CAD build for the part. Positions are in the model's coordinates, mm. A direction names the side the tool comes from. Give positions to 0.01 mm unless a question says otherwise; leave off trailing zeros. Loops run counter-clockwise (first coordinate to the right, second up) from the corner with the lowest first, then second, coordinate; pieces in that order, holes last. Notation, with made-up numbers: (-22.5, 24.5) -> (-1.5, 24.5) arc R25 cw to (-1.5, 50.5) -> close; hole circle Ø2 at (9, 82.5). An arc over 180 degrees is marked (long way). Write each question's results on one line, items separated by ' | '. Start each with the question number.
Autodesk Inventor part; units mm, degrees
ref_plane "YZ Plane" through (0, 0, 0) normal (1, 0, 0) x (0, 1, 0)
ref_plane "XZ Plane" through (0, 0, 0) normal (0, 1, 0) x (-1, 0, 0)
ref_plane "XY Plane" through (0, 0, 0) normal (0, 0, 1) x (1, 0, 0)
sketch "Sketch1" plane through (0, 0, 0) normal (0, 1, 0) x (-1, 0, 0)
  line L0 (22.75, -10.36) -> (7.75, -10.36)
  line L1 (7.75, -10.36) -> (-0.1031, 0)
  circle A0 centre (4.34, -10.36) radius 1
  line L2 (22.75, 10.36) -> (7.75, 10.36)
  circle A1 centre (12.64, 0) radius 9.6 construction
  line L3 (22.75, 12.36) -> (22.75, -12.36)
  circle A2 centre (4.34, 10.36) radius 1
  line L4 (7.75, 10.36) -> (-0.1031, 0)
  line L5 (26.25, 19) -> (26.25, -19)
  line L6 (22.75, -12.36) -> (-22.75, -12.36)
  line L7 (22.75, 0) -> (-22.75, 0) construction
  line L8 (26.25, -19) -> (-28.75, -19)
  line L9 (26.25, -19) -> (-28.75, 19) construction
  line L10 (-28.75, -19) -> (26.25, 19) construction
  line L11 (-22.75, 12.36) -> (22.75, 12.36)
  line L12 (-28.75, 19) -> (26.25, 19)
  line L13 (-28.75, -19) -> (-28.75, 19)
  circle A3 centre (-16.36, 10.25) radius 1
  line L14 (-22.75, -12.36) -> (-22.75, 12.36)
  circle A4 centre (-16.36, -10.25) radius 1
  point P0 (0, 0)
  point P1 (-1.25, 0)
  point P2 (0, 0)
  point P3 (22.75, -10.36)
  dimension "d0" = 55
  dimension "d1" = 38
  dimension "d2" = 45.5
  dimension "d3" = 24.72
  dimension "d4" = 2
  dimension "d6" = 18.41
  dimension "d7" = 20.5
  dimension "d8" = 19.2
  dimension "d9" = 10.11
  dimension "d10" = 13
  dimension "d11" = 15
  dimension "d12" = 3.5
  dimension "d13" = 2
  dimension "d14" = 3.41
  dimension "d66" = 20.7
extrude "Extrusion1" add sketch "Sketch1" along normal mid plane 1 contours L3 L6 L14 L11 L2 L4 L1 L0 | L5 L8 L13 L12
extrude "Extrusion2" add sketch "Sketch1" along normal blind 35 contours L5 L8 L13 L12
fillet "Fillet1" radius 3 8 edges at (1.25, -0.5, -19) (28.75, -0.5, 0) (1.25, -0.5, 19) (-26.25, -0.5, 0) (28.75, 17.25, -19) (28.75, 17.25, 19) (-26.25, 17.25, 19) (-26.25, 17.25, -19)
sketch "Sketch5" plane through (25.75, 2.5, -19) normal (0, 0, -1) x (-1, 0, 0)
  circle A0 centre (2.5, 14.75) radius 1.5
  circle A1 centre (2.5, 21.75) radius 1.5
  circle A2 centre (2.5, 28.75) radius 1.5
  circle A3 centre (16.5, 14.75) radius 1.5
  circle A4 centre (16.5, 21.75) radius 1.5
  circle A5 centre (16.5, 28.75) radius 1.5
  line L0 (-3, 32.5) -> (-3, 0)
  line L1 (0, 32.5) -> (49, 32.5)
  point P0 (25.75, -2.5)
  dimension "d47" = 3
  dimension "d52" = 7
  dimension "d55" = 14
  dimension "d67" = 3.75
  dimension "d68" = 5.5
hole "Hole2" at (23.25, 17.25, -19) at (23.25, 24.25, -19) at (9.25, 24.25, -19) at (9.25, 17.25, -19) at (23.25, 31.25, -19) at (9.25, 31.25, -19) direction (0, 0, 1) diameter 2.459 depth 6 tip angle 118 counterbore diameter 3.9 counterbore depth 3.8
sketch "Sketch8" plane through (0, 35, 0) normal (0, 1, 0) x (1, 0, 0)
  line L0 (-23.25, -19) -> (25.75, -19)
  line L1 (28.75, -16) -> (28.75, 16)
  point P0 (0, 0)
  point P1 (16.25, -15.68)
  dimension "d77" = 3.32
  dimension "d78" = 12.5
hole "Hole4" at (16.25, 35, 15.68) direction (0, -1, 0) diameter 2.459 depth 6 tip angle 118 counterbore diameter 3.9 counterbore depth 3.8
properties part number "basketlewy" material "PCTG 20%"
Q1. Which spindle directions (+Z, -Z, +X, -X, +Y, -Y) get a long thin tool onto all of the face, cutting with end or side? Do faces 1 (the face through (9.2, 22.3, -17.1)), 2 (the face through (22.75, 18, 0)), 3 (the face through (0.91, 0.36, 18.1)). Say none if no direction does.
Q2. Drop flat-ended pins along their axis: pin 1 (4.5 mm diameter, centred on x = 8.5, y = 17.5, fed in from -Z); pin 2 (6 mm diameter, centred on x = 9, z = 2, fed in from +Y); pin 3 (1.5 mm diameter, centred on x = 23.25, y = 24.25, fed in from -Z); pin 4 (1.9 mm diameter, centred on x = 23.5, y = 32, fed in from -Z). Give the stop position or say it passes through.
Q3. Mould opens along Y. For faces 4 (the face through (9.998, 30.274, -14.085)), 5 (the face through (7, -0.5, 0)), 6 (the face through (17.98, 33.07, 16.58)) say: pulls with the +Y half, pulls with the -Y half, needs draft (parallel to the pull), parting line crosses it, or undercut.
Q4. Wall check: L1, parallel to X at y = 31.25, z = -13.95; L2, parallel to Z at x = -15, y = 28; L3, parallel to Y at x = 9.25, z = -16. Give the ranges that are in metal, low to high.
Q5. Saw through at B-B, the plane y = 13.5. List the corners of the cut face in (x, z).
Q6. Saw through at C-C, the plane x = -9. List the corners of the cut face in (y, z).
Q7. Saw through at A-A, the plane x = 3. List the corners of the cut face in (y, z), then the cut area to 3 significant figures.
Q8. Saw through at D-D, the plane z = 8. List the corners of the cut face in (x, y), then the cut area to 3 significant figures.
Answer block:
1) face 1: -Z | face 2: +Y | face 3: +Z, +X, -X, -Y
2) pin 1: stops at z = -19 | pin 2: stops at y = 0.5 | pin 3: stops at z = -12.71 | pin 4: stops at z = -15.2
3) face 4: undercut | face 5: pulls with the -Y half | face 6: needs draft
4) L1: x = -26.25 to 8.02, 10.48 to 22.02, 24.48 to 28.75 | L2: z = -19 to -12.36, 12.36 to 19 | L3: y = -0.5 to 15.3, 19.2 to 22.3, 26.2 to 29.3, 33.2 to 35
5) outline: (-26.25, -16) arc R3 ccw to (-23.25, -19) -> (25.75, -19) arc R3 ccw to (28.75, -16) -> (28.75, 16) arc R3 ccw to (25.75, 19) -> (-23.25, 19) arc R3 ccw to (-26.25, 16) -> close; hole (-22.75, -12.36) -> (22.75, -12.36) -> (22.75, 12.36) -> (-22.75, 12.36) -> close
6) outline: (-0.5, -16) arc R3 ccw to (2.5, -19) -> (35, -19) -> (35, -12.36) -> (0.5, -12.36) -> (0.5, -10.36) -> (-0.5, -10.36) -> close; (-0.5, 10.36) -> (0.5, 10.36) -> (0.5, 12.36) -> (35, 12.36) -> (35, 19) -> (2.5, 19) arc R3 ccw to (-0.5, 16) -> close
7) outline: (-0.5, -16) arc R3 ccw to (2.5, -19) -> (35, -19) -> (35, -12.36) -> (0.5, -12.36) -> (0.5, 12.36) -> (35, 12.36) -> (35, 19) -> (2.5, 19) arc R3 ccw to (-0.5, 16) -> close | area: 492 mm2
8) outline: (-26.25, 2.5) arc R3 ccw to (-23.25, -0.5) -> (-22.75, -0.5) -> (-22.75, 35) -> (-26.25, 35) -> close; (-5.96, -0.5) -> (25.75, -0.5) arc R3 ccw to (28.75, 2.5) -> (28.75, 35) -> (22.75, 35) -> (22.75, 0.5) -> (-5.96, 0.5) -> close | area: 362 mm2
